Build history of the part. All positions in model axes, mm. A direction names the side the tool comes from. Coordinates: 2 decimals unless noted, no trailing zeros. Order: outer loops, then holes, each group sorted by start corner. A loop starts at its lowest first (then second) coordinate and runs counter-clockwise, first axis right, second up. Notation, with made-up numbers: (0, -8) - (19, -8) arc R16 ccw to (19, 20) - close; hole circle Ø6 at (-39, 4). An arc over 180 degrees is marked (long way). Answer as CSV lines item,"result". Start each with the question number.
from build123d import *

# Parameters (mm, degrees)
BOSS_EXTRUDE1_DEPTH = 3.175
SKETCH5_R           = 1.27
BOSS_EXTRUDE2_DEPTH = 5.08
SKETCH6_R           = 1.27
BOSS_EXTRUDE3_DEPTH = 5.08
SKETCH10_W          = 5.08
SKETCH10_H          = 16.51
BOSS_EXTRUDE6_DEPTH = 3.175


with BuildPart() as part:
    # Sketch2 → Boss-Extrude1 (new body)
    with BuildSketch(Plane(origin=(0, 0, 0), x_dir=(1, 0, 0), z_dir=(0, 1, 0))):
        with BuildLine():
            Line((-51.57005061, 3.080202438), (-0.770050609, 15.780202438))
            ThreePointArc((-0.770050609, 15.780202438), (0, 15.875), (0.770050609, 15.780202438))
            Line((0.770050609, 15.780202438), (51.57005061, 3.080202438))
            ThreePointArc((51.57005061, 3.080202438), (53.975, 0), (51.57005061, -3.080202438))
            Line((51.57005061, -3.080202438), (0.770050609, -15.780202438))
            ThreePointArc((0.770050609, -15.780202438), (0, -15.875), (-0.770050609, -15.780202438))
            Line((-0.770050609, -15.780202438), (-51.57005061, -3.080202438))
            ThreePointArc((-51.57005061, -3.080202438), (-53.975, 0), (-51.57005061, 3.080202438))
        make_face()
        Polygon((37.709139639, 0), (-0.307385689, -9.504131332), (-38.111149392, -0.065221488), (-0.294525174, 9.500916203), align=None, mode=Mode.SUBTRACT)
    extrude(amount=BOSS_EXTRUDE1_DEPTH)

    # Sketch5 → Boss-Extrude2 (add)
    with BuildSketch(Plane(origin=(0, 3.175, 0), x_dir=(1, 0, 0), z_dir=(0, 1, 0))):
        with Locations(Location((-50.8, 0, 0), (0, 0, 270))):
            Circle(SKETCH5_R)
    extrude(amount=BOSS_EXTRUDE2_DEPTH)

    # Sketch6 → Boss-Extrude3 (add)
    with BuildSketch(Plane(origin=(0, 3.175, 0), x_dir=(1, 0, 0), z_dir=(0, 1, 0))):
        with Locations(Location((50.8, 0, 0), (0, 0, 270))):
            Circle(SKETCH6_R)
    extrude(amount=BOSS_EXTRUDE3_DEPTH)

    # Sketch10 → Boss-Extrude6 (add)
    with BuildSketch(Plane(origin=(0, 3.175, 0), x_dir=(1, 0, 0), z_dir=(0, 1, 0))):
        with Locations((-15.24, 0)):
            Rectangle(SKETCH10_W, SKETCH10_H)
        with Locations((15.24, 0)):
            Rectangle(SKETCH10_W, SKETCH10_H)
    extrude(amount=-BOSS_EXTRUDE6_DEPTH)


solid = part.part
(1) Drop flat-ended pins along their axis: pin 1 Ø3.5 at (y, z) = (2.5, -2.5) entering from -X; pin 2 Ø1.5 at (x, z) = (18, -4) entering from +Y (3 decimals); pin 3 Ø2 at (y, z) = (3.5, 2.5) entering from +X. Give the stop position or say it passes through.
(2) Band-saw the part on B-B on z = -7.5. List the corners of the cut face in (x, y) (1 decimal), plus the area to 3 significant figures.
(3) Pull direction Z, two halves, no side cores. Call faces 1 (the flat face through (25.81, 1.57, -9.52)), 2 (the flat face through (6.287, 1.565, 7.855)), 3 (the cylindrical face through (49.56, 5.68, -0.28)): +Z half, -Z half, draft (parallel to the pull), parting line (faces both ways), or undercut.
(4) Band-saw the part on D-D on z = -12. List the corners of the cut face in (x, y) (3 decimals).
(5) Band-saw the part on C-C on x = 23. List the corners of the cut face in (y, z) (3 decimals).
(6) Which spindle directions (+Z, -Z, +X, -X, +Y, -Y) get a long thin tool onto all of the face, cutting with end or side? Do faces 4 (the flat face through (-6.58, 1.57, -7.91)), 5 (the flat face through (-26.53, 1.57, -9.34)). Say none if no direction does.
(7) Probe L1, parallel to Y at x = -19, z = -10.5 (3 decimals); L2, parallel to Z at x = 35, y = 2.5; L3, parallel to X at y = 5.5, z = 1. List the from-to ranges inside material, lowest first. Write a range as [from, to].
(8) Band-saw the part on A-A on y = 6.75. List the corners of the cut face in (x, z), plus the area to 3 significant figures.
Filled in:
1,pin 1,"stops at x = -53.89"
1,pin 2,"stops at y = 3.175"
1,pin 3,"stops at x = 53.57"
2,outline,"(-33.9, 0) - (-8.2, 0) - (-8.2, 3.2) - (-33.9, 3.2) - close; (7.7, 0) - (33.9, 0) - (33.9, 3.2) - (7.7, 3.2) - close"
2,area,"165 mm^2"
3,face 1,"-Z half"
3,face 2,"undercut"
3,face 3,"parting line"
4,outline,"(-15.891, 0) - (15.891, 0) - (15.891, 3.175) - (-15.891, 3.175) - close"
5,outline,"(0, -10.223) - (3.175, -10.223) - (3.175, -3.677) - (0, -3.677) - close; (0, 3.677) - (3.175, 3.677) - (3.175, 10.223) - (0, 10.223) - close"
6,face 4,"+Y, -Y"
6,face 5,"-Z, -X, +Y, -Y"
7,L1,"y = [0, 3.175]"
7,L2,"z = [-7.22, -0.68], [0.68, 7.22]"
7,L3,"x = [-51.58, -50.02], [50.02, 51.58]"
8,outline,"circle Ø2.54 at (-50.8, 0); circle Ø2.54 at (50.8, 0)"
8,area,"10.1 mm^2"
